from build123d import *

# Parameters (mm, degrees)
MODEL_W             = 70
MODEL_H             = 25
BOSS_EXTRUDE1_DEPTH = 3


with BuildPart() as part:
    # Model → Boss-Extrude1 (new body)
    with BuildSketch(Plane.XY):
        Polygon((249.402887008, 1.915275896), (249.402887008, -28.084724104), (252.402887008, -28.084724104), (252.402887008, -58.084724104), (180.402887008, -58.084724104), (180.402887008, -57.084724104), (150.402887008, -57.084724104), (150.402887008, -58.084724104), (78.402887008, -58.084724104), (78.402887008, -28.084724104), (81.402887008, -28.084724104), (81.402887008, 1.915275896), (78.402887008, 1.915275896), (78.402887008, 31.915275896), (89.402887008, 31.915275896), (89.402887008, 28.915275896), (99.402887008, 28.915275896), (99.402887008, 31.915275896), (160.402887008, 31.915275896), (160.402887008, 28.915275896), (170.402887008, 28.915275896), (170.402887008, 31.915275896), (231.402887008, 31.915275896), (231.402887008, 28.915275896), (241.402887008, 28.915275896), (241.402887008, 31.915275896), (252.402887008, 31.915275896), (252.402887008, 1.915275896), align=None)
        with Locations((149.402887008, -25.584724104)):
            Rectangle(MODEL_W, MODEL_H, mode=Mode.SUBTRACT)
    extrude(amount=BOSS_EXTRUDE1_DEPTH)


solid = part.part
Can you work these out from the model? Positions are in its coordinate system, mm. A direction names the side the tool comes from. Give positions to 0.01 mm unless a question says otherwise; leave off trailing zeros. Loops run counter-clockwise (first coordinate to the right, second up) from the corner with the lowest first, then second, coordinate; pieces in that order, holes last. Notation, with made-up numbers: (54, 12.5) - (110, 12.5) arc R18 ccw to (110, 32.5) - close; hole circle Ø1 at (17, 83.5). An arc over 180 degrees is marked (long way). Return JSON: item names as keys, results as strings.
1. If I drill on line 1 (X direction, y = -36, z = 2.8); line 2 (Y direction, x = 140, z = 2.55); line 3 (Y direction, x = 167.5, z = 2.7), over which ranges is the centre line in solid material (lowest first)?
Output values:
{"line 1": "x = 78.4 to 114.4, 184.4 to 252.4", "line 2": "y = -58.08 to -38.08, -13.08 to 31.92", "line 3": "y = -57.08 to -38.08, -13.08 to 28.92"}
2. I want a section at B-B on y = -35. Please give me the cut outline in (x, z), and give its area (3 significant figures).
Output values:
{"outline": "(78.4, 0) - (114.4, 0) - (114.4, 3) - (78.4, 3) - close; (184.4, 0) - (252.4, 0) - (252.4, 3) - (184.4, 3) - close", "area": "312 mm²"}
3. I want a section at A-A on x = 121.5. Please give me the cut outline in (y, z).
Output values:
{"outline": "(-58.08, 0) - (-38.08, 0) - (-38.08, 3) - (-58.08, 3) - close; (-13.08, 0) - (31.92, 0) - (31.92, 3) - (-13.08, 3) - close"}
4. For faces 1 (the face through (252.403, -43, 1)), 2 (the face through (80, 1.915, 1)), 3 (the face through (184.403, -26, 1)), 4 (the face through (89.403, 30, 1)), 5 (the face through (166, -57.085, 1)), which set-ups out of +Z, -Z, +X, -X, +Y, -Y let a thin tool reach every point of the face, with its end or its side?
Output values:
{"face 1": "+Z, -Z, +X, +Y, -Y", "face 2": "+Z, -Z, -X", "face 3": "+Z, -Z", "face 4": "+Z, -Z, +Y", "face 5": "+Z, -Z, -Y"}
5. We'd pull the mould along Y, two halves only. Please class faces 6 (the face through (80, -28.085, 1)), 7 (the face through (165, 28.915, 1)), 8 (the face through (115, -58.085, 1)): +Y half, -Y half, draft (parallel to the pull), parting line (faces both ways), or undercut.
Output values:
{"face 6": "undercut", "face 7": "+Y half", "face 8": "-Y half"}
6. I'm going to push flat-ended pins straight in: pin 1 Ø0.9 at (x, z) = (93.5, 1.5) entering from +Y; pin 2 Ø1.5 at (y, z) = (-19.5, 1.5) entering from -X. Where does each tip first touch, or does it pass through?
Output values:
{"pin 1": "stops at y = 28.92", "pin 2": "stops at x = 81.4"}
7. I want a section at D-D on y = 0. Please give me the cut outline in (x, z), and give its area (3 significant figures).
Output values:
{"outline": "(81.4, 0) - (249.4, 0) - (249.4, 3) - (81.4, 3) - close", "area": "504 mm²"}
